from build123d import *

# Parameters (mm, degrees)
F0_R     = 16
F1_DEPTH = 1
F2_R     = 8.5
F3_DEPTH = 2
F4_R     = 5.75
F5_DEPTH = 10
F7_DEPTH = 10


with BuildPart() as f1:
    # F0 (on Top) → F1 (new body)
    with BuildSketch(Plane.XY):
        Circle(F0_R)
    extrude(amount=F1_DEPTH)

    # F2 (on face) → F3 (join)
    with BuildSketch(Plane.XY.offset(1)):
        Circle(F2_R)
    extrude(amount=F3_DEPTH)

    # F4 (on face) → F5 (join)
    with BuildSketch(Plane.XY.offset(3)):
        Circle(F4_R)
    extrude(amount=F5_DEPTH)

    # F6 (on face) → F7 (cut)
    with BuildSketch(Plane.XY.offset(13)):
        with BuildLine():
            Line((0, 1), (0, 5.75))
            ThreePointArc((0, 5.75), (-4.25, 3.872983), (-5.72528, -0.532609))
            Line((-5.72528, -0.532609), (-0.995701, -0.092628))
            ThreePointArc((-0.995701, -0.092628), (-0.673562, -0.73913), (0, -1))
            Line((0, -1), (0, -5.75))
            ThreePointArc((0, -5.75), (4.25, -3.872983), (5.72528, 0.532609))
            Line((5.72528, 0.532609), (0.995701, 0.092628))
            ThreePointArc((0.995701, 0.092628), (0.673562, 0.73913), (0, 1))
        make_face()
    extrude(amount=-F7_DEPTH, mode=Mode.SUBTRACT)


solid = f1.part
Design review of the part built by this model. Coordinates are the model's own, in mm. A direction names the side the tool comes from. Round coordinates to 2 decimals unless told otherwise and drop trailing zeros. Write each loop counter-clockwise with the first axis right and the second up, starting at its lowest first coordinate (ties: lowest second). Pieces come first, ordered by that corner, then holes.
Item 1: For faces 1 (the flat face through (-3.394, -0.316, 8.07)), 2 (the flat face through (7, -7, 1)), 3 (the cylindrical face through (-3.917, -4.21, 7.93)), 4 (the cylindrical face through (3.917, 4.21, 7.93)), 5 (the flat face through (0, -3, 8)), list the 3-axis set-ups (+Z, -Z, +X, -X, +Y, -Y) from which the entire face can be reached by the end or side of a thin tool; tool diameter is ignored.
Item 2: Consider section D-D on y = 6.5. Give the boundary of the cut face in (x, z).
Item 3: Wall thickness on L1, parallel to Z at x = 8.5, y = 10.5; L2, parallel to Y at x = 4, z = 9.75; L3, parallel to X at y = 5, z = 6: over which ranges is each line inside the solid? List them lowest first.
Item 4: For pin 1 Ø2 at (x, z) = (-5.5, 9) entering from -Y; pin 2 Ø5 at (y, z) = (-4.5, 10.5) entering from +X; pin 3 Ø1.4 at (y, z) = (3, 6) entering from -X, all flat-tipped, find the tip position at first contact; note any pin that passes through.
Item 5: Consider section B-B on y = 1.5. Give the boundary of the cut face in (x, z).
Item 6: Consider section C-C on x = -2.5. Give the boundary of the cut face in (y, z), and give its area (3 significant figures).
Item 7: Consider section A-A on z = 7. Give the boundary of the cut face in (x, y), and give its area (3 significant figures).
Check values:
1. face 1: +Z, -X, +Y
1. face 2: +Z
1. face 3: +Z, -X, -Y
1. face 4: +Z, +X, +Y
1. face 5: +Z, +X, -Y
2. outline: (-14.62, 0) - (14.62, 0) - (14.62, 1) - (5.48, 1) - (5.48, 3) - (-5.48, 3) - (-5.48, 1) - (-14.62, 1) - close
3. L1: z = 0 to 1
3. L2: y = 0.37 to 4.13
3. L3: x = 0 to 2.84
4. pin 1: stops at y = -3.58
4. pin 2: stops at x = 0
4. pin 3: stops at x = 0
5. outline: (-15.93, 0) - (15.93, 0) - (15.93, 1) - (8.37, 1) - (8.37, 3) - (5.55, 3) - (5.55, 13) - (0, 13) - (0, 3) - (-8.37, 3) - (-8.37, 1) - (-15.93, 1) - close
6. outline: (-15.8, 0) - (15.8, 0) - (15.8, 1) - (8.12, 1) - (8.12, 3) - (-0.23, 3) - (-0.23, 13) - (-5.18, 13) - (-5.18, 3) - (-8.12, 3) - (-8.12, 1) - (-15.8, 1) - close
6. area: 114 mm2
7. outline: (-5.73, -0.53) arc R5.75 ccw to (0, -5.75) - (0, -1) arc R1 cw to (-1, -0.09) - close; (0, 1) arc R1 cw to (1, 0.09) - (5.73, 0.53) arc R5.75 ccw to (0, 5.75) - close
7. area: 47.4 mm2
